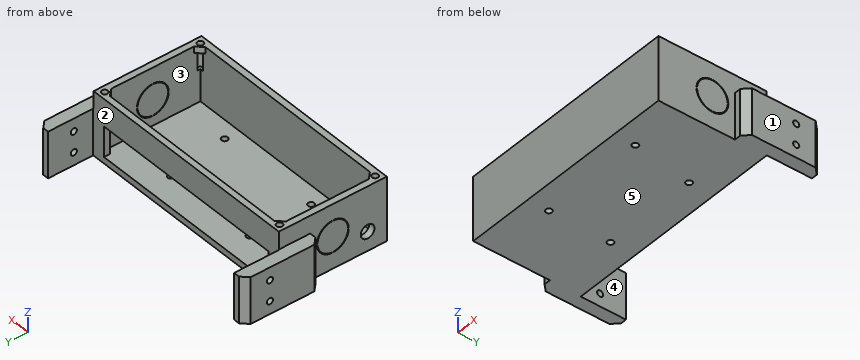
from build123d import *

# Parameters (mm, degrees)
SKETCH1_W           = 177
SKETCH1_H           = 85
BOSS_EXTRUDE1_DEPTH = 50
SHELL1_T            = -5
SKETCH2_W           = 157.4
SKETCH2_H           = 23.7
CUT_EXTRUDE1_DEPTH  = 6
SKETCH4_R           = 5.375
CUT_EXTRUDE2_DEPTH  = 6
SKETCH6_R           = 2.375
BOSS_EXTRUDE3_DEPTH = 5
SKETCH7_R           = 2.375
CUT_EXTRUDE4_DEPTH  = 20
SKETCH8_W           = 10
SKETCH8_H           = 60
BOSS_EXTRUDE4_DEPTH = 36.2
CHAMFER1_SIZE       = 5
SKETCH9_W           = 177.8
SKETCH9_H           = 35.8
SKETCH9_W_2         = 177
SKETCH9_H_2         = 35
CUT_EXTRUDE5_DEPTH  = 51
SKETCH10_R          = 2.4
CUT_EXTRUDE6_DEPTH  = 198
SKETCH11_R          = 2.4
CUT_EXTRUDE8_DEPTH  = 5
CUT_EXTRUDE14_DEPTH = 188


with BuildPart() as part:
    # Sketch1 → Boss-Extrude1 (new body)
    with BuildSketch(Plane.XY):
        Rectangle(SKETCH1_W, SKETCH1_H)
    extrude(amount=BOSS_EXTRUDE1_DEPTH)

    # Shell1
    shell1_openings = [part.faces().sort_by_distance(p)[0] for p in [
        (0, 0, 50),
    ]]
    offset(amount=SHELL1_T, openings=shell1_openings, kind=Kind.INTERSECTION)

    # Sketch2 → Cut-Extrude1 (cut, through all)
    with BuildSketch(Plane.XZ.offset(-37.5)):
        with Locations((0, 16.85)):
            Rectangle(SKETCH2_W, SKETCH2_H)
    extrude(amount=-CUT_EXTRUDE1_DEPTH, mode=Mode.SUBTRACT)

    # Sketch4 → Cut-Extrude2 (cut, through all)
    with BuildSketch(Plane(origin=(-83.5, 0, 0), x_dir=(0, 0, -1), z_dir=(1, 0, 0))):
        with Locations((-15, -27.5)):
            Circle(SKETCH4_R)
    extrude(amount=-CUT_EXTRUDE2_DEPTH, mode=Mode.SUBTRACT)

    # Sketch6 → Boss-Extrude3 (add)
    with BuildSketch(Plane.XY.offset(50)):
        Polygon((87.009300393, 41.009300393), (75.027799397, 41.009300393), (87.009300393, 29.027799397), align=None)
        with Locations((83.5, 37.5)):
            Circle(SKETCH6_R, mode=Mode.SUBTRACT)
        Polygon((75.027799397, -41.009300393), (87.009300393, -29.027799397), (87.009300393, -41.009300393), align=None)
        with Locations((83.5, -37.5)):
            Circle(SKETCH6_R, mode=Mode.SUBTRACT)
        Polygon((-87.009300393, -41.009300393), (-75.027799397, -41.009300393), (-87.009300393, -29.027799397), align=None)
        with Locations((-83.5, -37.5)):
            Circle(SKETCH6_R, mode=Mode.SUBTRACT)
        Polygon((-75.027799397, 41.009300393), (-87.009300393, 29.027799397), (-87.009300393, 41.009300393), align=None)
        with Locations((-83.5, 37.5)):
            Circle(SKETCH6_R, mode=Mode.SUBTRACT)
    extrude(amount=-BOSS_EXTRUDE3_DEPTH)

    # Sketch7 → Cut-Extrude4 (cut)
    with BuildSketch(Plane.XY.offset(50)):
        with Locations((83.5, 37.5)):
            Circle(SKETCH7_R)
        with Locations((83.5, -37.5)):
            Circle(SKETCH7_R)
        with Locations((-83.5, -37.5)):
            Circle(SKETCH7_R)
        with Locations((-83.5, 37.5)):
            Circle(SKETCH7_R)
    extrude(amount=-CUT_EXTRUDE4_DEPTH, mode=Mode.SUBTRACT)

    # Sketch8 → Boss-Extrude4 (add)
    with BuildSketch(Plane(origin=(0, 0, 0), x_dir=(-1, 0, 0), z_dir=(0, 0, -1))):
        with Locations((-93.5, 47.5)):
            Rectangle(SKETCH8_W, SKETCH8_H)
        with Locations((93.5, 47.5)):
            Rectangle(SKETCH8_W, SKETCH8_H)
    extrude(amount=-BOSS_EXTRUDE4_DEPTH)

    # Chamfer1
    chamfer1_edges = [part.edges().sort_by_distance(p)[0] for p in [
        (98.5, 17.5, 18.1),
        (98.5, 77.5, 18.1),
        (-98.5, 77.5, 18.1),
        (-98.5, 17.5, 18.1),
    ]]
    chamfer(chamfer1_edges, length=CHAMFER1_SIZE)

    # Sketch9 → Cut-Extrude5 (cut, through all)
    with BuildSketch(Plane(origin=(0, 0, 0), x_dir=(-1, 0, 0), z_dir=(0, 0, -1))):
        with Locations((0, 60)):
            Rectangle(SKETCH9_W, SKETCH9_H)
        with Locations((0, 60)):
            Rectangle(SKETCH9_W_2, SKETCH9_H_2, mode=Mode.SUBTRACT)
    extrude(amount=-CUT_EXTRUDE5_DEPTH, mode=Mode.SUBTRACT)

    # Sketch10 → Cut-Extrude6 (cut, through all)
    with BuildSketch(Plane(origin=(-98.5, 0, 0), x_dir=(0, 0, -1), z_dir=(1, 0, 0))):
        with Locations((-26.2, 57.3)):
            Circle(SKETCH10_R)
        with Locations((-10, 57.3)):
            Circle(SKETCH10_R)
    extrude(amount=CUT_EXTRUDE6_DEPTH, mode=Mode.SUBTRACT)

    # Sketch11 → Cut-Extrude8 (cut)
    with BuildSketch(Plane.XY.offset(5)):
        with Locations((45.9486, -25.738739303)):
            Circle(SKETCH11_R)
        with Locations((38.4556, 22.597460697)):
            Circle(SKETCH11_R)
        with Locations((-36.6776, 22.597460697)):
            Circle(SKETCH11_R)
        with Locations((-36.6776, -25.738739303)):
            Circle(SKETCH11_R)
    extrude(amount=-CUT_EXTRUDE8_DEPTH, mode=Mode.SUBTRACT)

    # Sketch12 → Cut-Extrude14 (cut, through all)
    with BuildSketch(Plane.ZY.offset(88.5)):
        with BuildLine():
            Line((24.5, 11.789578808), (24.5, 12.289995997))
            ThreePointArc((24.5, 12.289995997), (16.161165235, 8.638834765), (12.510004003, 0.3))
            Line((12.510004003, 0.3), (13.010421192, 0.3))
            ThreePointArc((13.010421192, 0.3), (16.514718626, 8.285281374), (24.5, 11.789578808))
        make_face()
        with BuildLine():
            Line((13.010421192, -0.7), (12.510004003, -0.7))
            ThreePointArc((12.510004003, -0.7), (16.161165235, -9.038834765), (24.5, -12.689995997))
            Line((24.5, -12.689995997), (24.5, -12.189578808))
            ThreePointArc((24.5, -12.189578808), (16.514718626, -8.685281374), (13.010421192, -0.7))
        make_face()
        with BuildLine():
            Line((37.489995997, -0.7), (36.989578808, -0.7))
            ThreePointArc((36.989578808, -0.7), (33.485281374, -8.685281374), (25.5, -12.189578808))
            Line((25.5, -12.189578808), (25.5, -12.689995997))
            ThreePointArc((25.5, -12.689995997), (33.838834765, -9.038834765), (37.489995997, -0.7))
        make_face()
        with BuildLine():
            ThreePointArc((37.489995997, 0.3), (33.838834765, 8.638834765), (25.5, 12.289995997))
            Line((25.5, 12.289995997), (25.5, 11.789578808))
            ThreePointArc((25.5, 11.789578808), (33.485281374, 8.285281374), (36.989578808, 0.3))
            Line((36.989578808, 0.3), (37.489995997, 0.3))
        make_face()
    extrude(amount=-CUT_EXTRUDE14_DEPTH, mode=Mode.SUBTRACT)


solid = part.part
Part model, mm, in its own coordinate system. Face numbers are marked on the shaded views. A direction names the side the tool comes from. Coordinates: 2 decimals unless noted, no trailing zeros. Loops run counter-clockwise (first coordinate to the right, second up) from the corner with the lowest first, then second, coordinate; pieces in that order, holes last. Notation, with made-up numbers: (-26.75, 18) -> (14.25, 18) arc R22 ccw to (14.25, 57) -> close; hole circle Ø2 at (87.5, 30.25). An arc over 180 degrees is marked (long way). Use a Markdown table: item, result. Add a question column.
Item 1: Band-saw the part on C-C on y = 28.5. Write the cut outline in (x, z).
Item 2: Flat gauge pins, fed straight in: P1, Ø8.5, axis at y = -27.5, z = 15, coming from the +X side; P2, Ø13.5, axis at y = 15.5, z = 24.5, coming from the +X side; P3, Ø4, axis at x = 83.5, y = -37.5, coming from the +Z side; P4, Ø11, axis at x = 93, y = 40, coming from the +Z side. Where does each tip first touch, or does it go through?
Item 3: Probe probe 1 along Z at (x, y) = (-85, -27); probe 2 along X at (y, z) = (5, 13.5); probe 3 along Y at (x, z) = (80, 11). List the from-to ranges inside material, lowest first.
Item 4: Which spindle directions (+Z, -Z, +X, -X, +Y, -Y) get a long thin tool onto all of the face, cutting with end or side? Do the marked faces 4 and 5. Say none if no direction does.
Item 5: Pull direction Y, two halves, no side cores. Call the marked faces 1, 2 and 3: +Y half, -Y half, draft (parallel to the pull), parting line (faces both ways), or undercut.
Item 6: Band-saw the part on D-D on z = 15. Give the number of separate pieces and of enclosed holes in the cut face, plus the area to 3 significant figures.
Item 7: Band-saw the part on B-B on x = 73. Write the cut outline in (y, z), plus the area to 3 significant figures.
Item 8: Band-saw the part on A-A on z = 40. Write the cut outline in (x, y) (3 decimals), plus the area to 3 significant figures.
Geometry says:
| question | item | result |
|---|---|---|
| 1 | outline | (-98.5, 0) -> (98.5, 0) -> (98.5, 36.2) -> (88.5, 36.2) -> (88.5, 50) -> (83.5, 50) -> (83.5, 5) -> (-83.5, 5) -> (-83.5, 50) -> (-88.5, 50) -> (-88.5, 36.2) -> (-98.5, 36.2) -> close |
| 2 | P1 | x = 88.5 |
| 2 | P2 | x = 98.25 |
| 2 | P3 | z = 30 |
| 2 | P4 | z = 50 |
| 3 | probe 1 | 0 to 9.65, 20.35 to 50 |
| 3 | probe 2 | -88.5 to -83.5, 83.5 to 88.5 |
| 3 | probe 3 | -42.5 to -37.5, 37.5 to 42.1 |
| 4 | face 4 | +Z, -Z, +Y |
| 4 | face 5 | -Z, +X, -X, +Y, -Y |
| 5 | face 1 | draft |
| 5 | face 2 | +Y half |
| 5 | face 3 | undercut |
| 6 | separate pieces | 6 |
| 6 | enclosed holes | 0 |
| 6 | area | 2,780 mm² |
| 7 | outline | (-42.5, 0) -> (42.1, 0) -> (42.1, 5) -> (-37.5, 5) -> (-37.5, 50) -> (-42.5, 50) -> close; (37.5, 28.7) -> (42.1, 28.7) -> (42.1, 50) -> (37.5, 50) -> close |
| 7 | area | 746 mm² |
| 8 | outline | (-88.5, -42.5) -> (88.5, -42.5) -> (88.5, 42.1) -> (-88.5, 42.1) -> close; hole (-83.5, -35.125) arc R2.375 ccw (long way) to (-81.125, -37.5) -> (81.125, -37.5) arc R2.375 ccw (long way) to (83.5, -35.125) -> (83.5, 35.125) arc R2.375 ccw (long way) to (81.125, 37.5) -> (-81.125, 37.5) arc R2.375 ccw (long way) to (-83.5, 35.125) -> close |
| 8 | area | 2,400 mm² |
